Read the model definition and answer for the solid it produces. Units are mm, in the model's axes. A direction names the side the tool comes from. Coordinates: 2 decimals unless noted, no trailing zeros. Loops run counter-clockwise (first coordinate to the right, second up) from the corner with the lowest first, then second, coordinate; pieces in that order, holes last.
from build123d import *

# Parameters (mm, degrees)
BOSS_EXTRUDE2_DEPTH = 6.35
SKETCH4_R           = 3.175
CUT_EXTRUDE1_DEPTH  = 12.7
CUT_EXTRUDE2_DEPTH  = 2.032


with BuildPart() as part:
    # Sketch3 → Boss-Extrude2 (new body)
    with BuildSketch(Plane(origin=(0, 0, 0), x_dir=(1, 0, 0), z_dir=(0, 1, 0))):
        with BuildLine():
            Line((-17.4625, 6.35), (17.4625, 6.35))
            ThreePointArc((17.4625, 6.35), (18.581211108, 0), (17.4625, -6.35))
            Line((17.4625, -6.35), (-17.4625, -6.35))
            ThreePointArc((-17.4625, -6.35), (-18.581211108, 0), (-17.4625, 6.35))
        make_face()
    extrude(amount=BOSS_EXTRUDE2_DEPTH)

    # Sketch4 → Cut-Extrude1 (cut)
    with BuildSketch(Plane(origin=(0, 6.35, 0), x_dir=(1, 0, 0), z_dir=(0, 1, 0))):
        with Locations((13.335, 0)):
            Circle(SKETCH4_R)
        with Locations((-13.335, 0)):
            Circle(SKETCH4_R)
    extrude(amount=-CUT_EXTRUDE1_DEPTH, mode=Mode.SUBTRACT)

    # Sketch5 → Cut-Extrude2 (cut)
    with BuildSketch(Plane.XZ):
        with BuildLine():
            Line((17.4625, 6.35), (-4.1275, 6.35))
            Line((-4.1275, 6.35), (-4.1275, -6.35))
            Line((-4.1275, -6.35), (17.4625, -6.35))
            ThreePointArc((17.4625, -6.35), (18.581211108, 0), (17.4625, 6.35))
        make_face()
    extrude(amount=-CUT_EXTRUDE2_DEPTH, mode=Mode.SUBTRACT)


solid = part.part
Item 1: Given pin 1 (1.5 mm diameter, centred on y = 1, z = 3.5, fed in from -X); pin 2 (4 mm diameter, centred on x = 10, z = -0.5, fed in from -Y); pin 3 (1 mm diameter, centred on y = 0.5, z = -2.5, fed in from +X), each flat-ended and moving along its own axis, determine where each tip first touches the part or whether it passes through.
Numbers:
pin 1: stops at x = -18.38
pin 2: stops at y = 2.03
pin 3: stops at x = -4.13
Item 2: A cutting plane is placed at D-D on z = 1.75. Determine the outline of the cut face in (x, y), then the cut area to 3 significant figures.
Numbers:
outline: (-18.5, 0) - (-15.98, 0) - (-15.98, 6.35) - (-18.5, 6.35) - close; (-10.69, 0) - (-4.13, 0) - (-4.13, 2.03) - (10.69, 2.03) - (10.69, 6.35) - (-10.69, 6.35) - close; (15.98, 2.03) - (18.5, 2.03) - (18.5, 6.35) - (15.98, 6.35) - close
area: 132 mm2
Item 3: A cutting plane is placed at A-A on z = 0. Determine the outline of the cut face in (x, y), then the cut area to 3 significant figures.
Numbers:
outline: (-18.58, 0) - (-16.51, 0) - (-16.51, 6.35) - (-18.58, 6.35) - close; (-10.16, 0) - (-4.13, 0) - (-4.13, 2.03) - (10.16, 2.03) - (10.16, 6.35) - (-10.16, 6.35) - close; (16.51, 2.03) - (18.58, 2.03) - (18.58, 6.35) - (16.51, 6.35) - close
area: 122 mm2
Item 4: A cutting plane is placed at C-C on y = 5.75. Give the number of separate pieces and of enclosed holes in the cut face, then the cut area to 3 significant figures.
Numbers:
separate pieces: 1
enclosed holes: 2
area: 399 mm2
Item 5: A cutting plane is placed at B-B on x = -14.5. Determine the outline of the cut face in (y, z), then the cut area to 3 significant figures.
Numbers:
outline: (0, -6.35) - (6.35, -6.35) - (6.35, -2.95) - (0, -2.95) - close; (0, 2.95) - (6.35, 2.95) - (6.35, 6.35) - (0, 6.35) - close
area: 43.1 mm2
Item 6: Find the intervals of material crossed by line 1 along X through (y, z) = (2.75, 1); line 2 along X through (y, z) = (2.75, -0.5); line 3 along Y through (x, z) = (8.5, -4), in increasing order.
Numbers:
line 1: x = -18.55 to -16.35, -10.32 to 10.32, 16.35 to 18.55
line 2: x = -18.57 to -16.47, -10.2 to 10.2, 16.47 to 18.57
line 3: y = 2.03 to 6.35
Item 7: Which of the six approach directions +Z, -Z, +X, -X, +Y, -Y give full straight-line access (tool end or side, diameter ignored) to faces 1 (the face through (7, 2.032, 0)), 2 (the face through (18.58, 4.16, -0.09))?
Numbers:
face 1: +Z, -Z, +X, -Y
face 2: +X, +Y, -Y
Item 8: Determine the mould class of faces 3 (the face through (-10.307, 3.219, -0.954)), 4 (the face through (10.815, 4.221, 1.932)), 5 (the face through (-4.128, 1, 0)), 6 (the face through (0, 4, 6.35)) for opening direction Z: released by +Z, released by -Z, zero draft, split by the parting line, or undercut.
Numbers:
face 3: undercut
face 4: undercut
face 5: zero draft
face 6: released by +Z
